```python
from build123d import *

# Parameters (mm, degrees)
F1_DEPTH = 63.5
F0_W     = 22.195993
F0_H     = 19.05
F2_DEPTH = 25.4
F3_DEPTH = 7.9375
F0_W_2   = 25.4
F0_H_2   = 28.575


with BuildPart() as f1:
    # F0 (on Front) → F1 (new body, symmetric)
    with BuildSketch(Plane.XZ):
        Polygon((41.275, -9.525), (41.275, 9.525), (22.225, 9.525), (-41.275, 9.525), (-41.275, -9.525), align=None)
    extrude(amount=F1_DEPTH, both=True)

    # F0 (on Front) → F2 (join, symmetric)
    with BuildSketch(Plane.XZ):
        with BuildLine():
            Line((22.225, 9.525), (41.275, 9.525))
            Line((41.275, 9.525), (41.275, 27.0002))
            ThreePointArc((41.275, 27.0002), (45.92468, 38.22552), (57.15, 42.8752))
            Line((57.15, 42.8752), (60.325, 42.8752))
            Line((60.325, 42.8752), (60.325, 61.9252))
            Line((60.325, 61.9252), (57.15, 61.9252))
            ThreePointArc((57.15, 61.9252), (32.454296, 51.695904), (22.225, 27.0002))
            Line((22.225, 27.0002), (22.225, 9.525))
        make_face()
        with Locations((71.422996, 52.4002)):
            Rectangle(F0_W, F0_H)
    extrude(amount=F2_DEPTH, both=True)

    # F0 (on Front) → F3 (join, symmetric)
    with BuildSketch(Plane.XZ):
        with BuildLine():
            Line((-41.275, 9.525), (22.225, 9.525))
            Line((22.225, 9.525), (22.225, 27.0002))
            ThreePointArc((22.225, 27.0002), (32.454296, 51.695904), (57.15, 61.9252))
            add(Edge.make_bspline(
                [(-41.275, 9.525), (-41.22147, 31.626377), (27.588112, 61.989266), (57.15, 61.9252)],
                knots=[0, 0, 0, 0, 111.504536, 111.504536, 111.504536, 111.504536], degree=3))
        make_face()
    extrude(amount=F3_DEPTH, both=True)

    # F0 (on Front) → F4 (revolve)
    with BuildSketch(Plane.XZ):
        with Locations((98.425, 52.3875)):
            Rectangle(F0_W_2, F0_H_2)
    revolve(axis=Axis((85.725, 0, 52.3875), (0, 0, -1)))


solid = f1.part
```
Verification items for the finished model (mm, model axes). A direction names the side the tool comes from. Coordinates: 2 decimals unless noted, no trailing zeros. Loops run counter-clockwise (first coordinate to the right, second up) from the corner with the lowest first, then second, coordinate; pieces in that order, holes last. Notation, with made-up numbers: (-12.5, -7) - (45.5, -7) arc R25 ccw to (45.5, 17) - close; hole circle Ø1 at (24.5, 80). An arc over 180 degrees is marked (long way). Return JSON: item names as keys, results as strings.
1. Section check B-B, the plane x = 96. Record the boundary of the cut face in (y, z) (3 decimals), then the cut area to 3 significant figures.
Established:
{"outline": "(-23.229, 38.1) - (23.229, 38.1) - (23.229, 66.675) - (-23.229, 66.675) - close", "area": "1,330 mm2"}
2. Tool access check on faces 1 (the flat face through (45, 25.4, 42)), 2 (the cylindrical face through (32.73, -16.79, 51.97)), 3 (the flat face through (22.225, 17, 18)), 4 (the flat face through (45, -25.4, 42)). Record the directions out of +Z, -Z, +X, -X, +Y, -Y that give a thin tool (end or side, any length) a straight path to the whole face; none if there is none.
Established:
{"face 1": "+Z, +X, -X, +Y", "face 2": "+Z, -X, -Y", "face 3": "+Z, -X, +Y", "face 4": "+Z, +X, -X, -Y"}
3. Section check C-C, the plane y = 53. Record the boundary of the cut face in (x, z) (3 decimals), then the cut area to 3 significant figures.
Established:
{"outline": "(-41.275, -9.525) - (41.275, -9.525) - (41.275, 9.525) - (-41.275, 9.525) - close", "area": "1,570 mm2"}
4. Mould release check, pull along X, two halves, no side actions. Record for faces 5 (the flat face through (86, 0, 38.1)), 6 (the cylindrical face through (32.73, 16.55, 51.97)), 7 (the cylindrical face through (45.8, -0.4, 38.1)): +X half, -X half, draft (parallel to the pull), parting line (faces both ways), or undercut.
Established:
{"face 5": "draft", "face 6": "-X half", "face 7": "undercut"}
5. Section check A-A, the plane y = 23. Record the boundary of the cut face in (x, z) (3 decimals), then the cut area to 3 significant figures.
Established:
{"outline": "(-41.275, -9.525) - (41.275, -9.525) - (41.275, 27) arc R15.875 cw to (57.15, 42.875) - (74.947, 42.875) - (74.947, 38.1) - (96.503, 38.1) - (96.503, 66.675) - (74.947, 66.675) - (74.947, 61.925) - (57.15, 61.925) arc R34.925 ccw to (22.225, 27) - (22.225, 9.525) - (-41.275, 9.525) - close", "area": "3,620 mm2"}
6. Go/stop test with flat-tipped pins: pin 1 (8.5 mm diameter, centred on y = -14, z = 22, fed in from -X) (3 decimals); pin 2 (15.5 mm diameter, centred on x = 16.5, z = 28.5, fed in from -Y); pin 3 (18.5 mm diameter, centred on y = 31.5, z = 7, fed in from +X) (3 decimals). Record where each tip stops, or that it passes through.
Established:
{"pin 1": "stops at x = 22.225", "pin 2": "stops at y = -25.4", "pin 3": "stops at x = 41.275"}
7. Thickness scan on L1, parallel to X at y = 34, z = -1 (3 decimals); L2, parallel to Z at x = -17, y = 43.5 (3 decimals); L3, parallel to Y at x = 35.5, z = 20. Record the ranges inside material, lowest first.
Established:
{"L1": "x = -41.275 to 41.275", "L2": "z = -9.525 to 9.525", "L3": "y = -25.4 to 25.4"}
